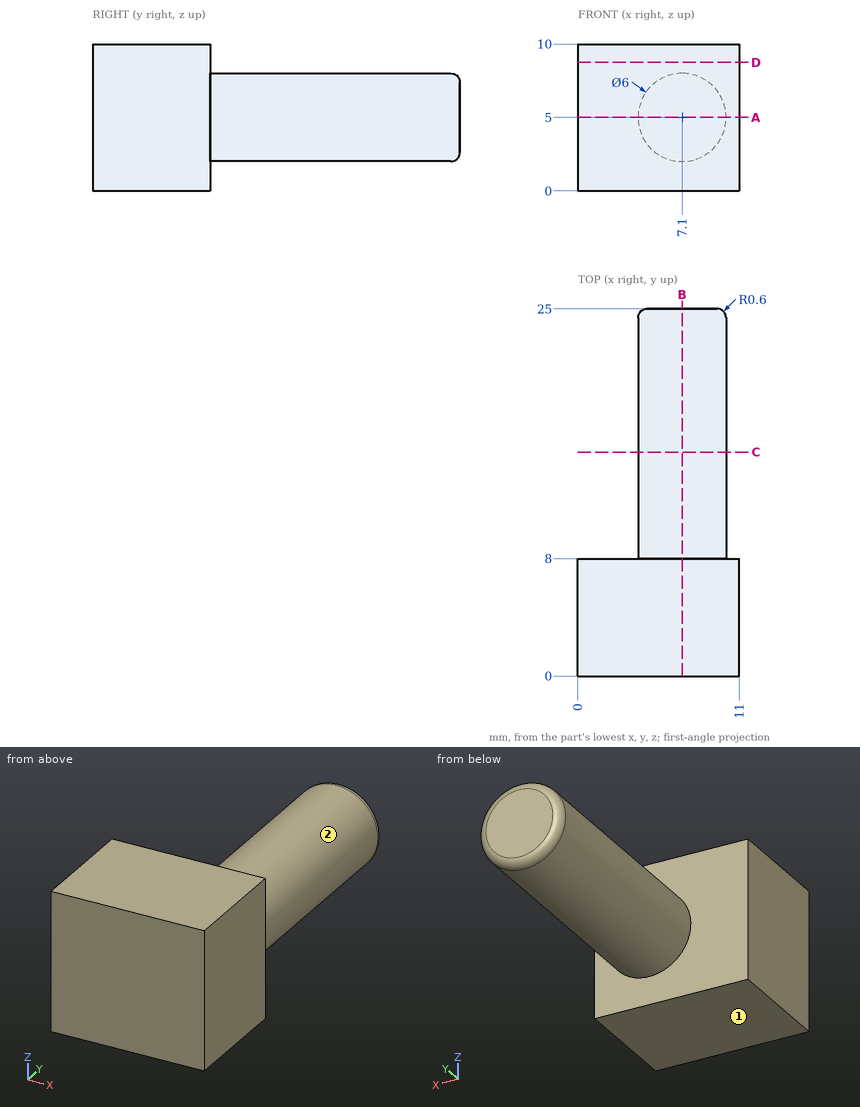
The drawing under review shows one solid part. Ordinate dimensions are in mm from its lowest x, y, z. A direction names the side the tool comes from. Coordinates: 2 decimals unless noted, no trailing zeros. Order: outer loops, then holes, each group sorted by start corner. A loop starts at its lowest first (then second) coordinate and runs counter-clockwise, first axis right, second up. Notation, with made-up numbers: (54.25, -25.5) -> (60.25, -25.5) arc R11 cw to (60.25, -12.5) -> close; hole circle Ø10 at (56.5, 64.5). An arc over 180 degrees is marked (long way). Answer in a Markdown table with one row per item.
(1) Machinability: for the marked faces 1 and 2, which of the approach directions +Z, -Z, +X, -X, +Y, -Y give a long, thin tool a straight path to every point of the face, cutting with its end or side? Answer none if there is none.
Answers:
| item | result |
|---|---|
| face 1 | -Z, +X, -X, +Y, -Y |
| face 2 | +Y |
(2) Consider section C-C (y = 15.25). Write out the cut boundary in (x, z).
Answers:
| item | result |
|---|---|
| outline | circle Ø6 at (7.1, 5) |
(3) Wall thickness on line 1 along Y through (x, z) = (3.25, 8); line 2 along Z through (x, y) = (7, 11.5); line 3 along X through (y, z) = (12.25, 7.25): over which ranges is each line inside the solid? List them lowest first.
Answers:
| item | result |
|---|---|
| line 1 | 0 to 8 |
| line 2 | 2 to 8 |
| line 3 | 5.12 to 9.08 |
(4) Consider section D-D (z = 8.75). Write out the cut boundary in (x, y).
Answers:
| item | result |
|---|---|
| outline | (0, 0) -> (11, 0) -> (11, 8) -> (0, 8) -> close |
(5) Consider section A-A (z = 5). Write out the cut boundary in (x, y), plus the area to 3 significant figures.
Answers:
| item | result |
|---|---|
| outline | (0, 0) -> (11, 0) -> (11, 8) -> (10.1, 8) -> (10.1, 24.4) arc R0.6 ccw to (9.5, 25) -> (4.7, 25) arc R0.6 ccw to (4.1, 24.4) -> (4.1, 8) -> (0, 8) -> close |
| area | 190 mm² |
(6) Insertion check: pin 1 (1 mm diameter, centred on y = 15.5, z = 4, fed in from -X). The pin has a flat end and moves straight along its axis. Give the tip position at first contact, or say it passes through.
Answers:
| item | result |
|---|---|
| pin 1 | x = 4.14 |
(7) Consider section B-B (x = 7.1). Write out the cut boundary in (y, z).
Answers:
| item | result |
|---|---|
| outline | (0, 0) -> (8, 0) -> (8, 2) -> (24.4, 2) arc R0.6 ccw to (25, 2.6) -> (25, 7.4) arc R0.6 ccw to (24.4, 8) -> (8, 8) -> (8, 10) -> (0, 10) -> close |
